from build123d import *

# Parameters (mm, degrees)
SKETCH001_R      = 2.5
PAD_DEPTH        = 10
HOLE_D           = 2.2
HOLE_DEPTH       = 25
HOLE_CBORE_D     = 4
HOLE_CBORE_DEPTH = 1.2


with BuildPart() as part:
    # Sketch001 → Pad (new body)
    with BuildSketch(Plane.XY):
        with BuildLine():
            Line((0, 0), (80, 0))
            Line((80, 0), (90, 5))
            Line((90, 5), (80, 10))
            Line((80, 10), (12.291288, 10))
            Line((12.291288, 5), (12.291288, 10))
            Line((2.5, 5), (12.291288, 5))
            ThreePointArc((2.291288, 6), (-2.447266, 4.489226), (2.5, 5))
            Line((11.291288, 6), (2.291288, 6))
            Line((11.291288, 10), (11.291288, 6))
            Line((0, 10), (11.291288, 10))
            ThreePointArc((0, 10), (-5, 5), (0, 0))
        make_face()
        with Locations((80, 5.087405)):
            Circle(SKETCH001_R, mode=Mode.SUBTRACT)
    extrude(amount=PAD_DEPTH)

    # Hole
    with Locations(Plane(origin=(0, 10, 0), x_dir=(-1, 0, 0), z_dir=(0, 1, 0))):
        with Locations((-6, 5)):
            CounterBoreHole(HOLE_D / 2, HOLE_CBORE_D / 2, HOLE_CBORE_DEPTH, depth=HOLE_DEPTH)


solid = part.part
Part model, mm, in its own coordinate system. A direction names the side the tool comes from. Give positions to 0.01 mm unless a question says otherwise; leave off trailing zeros. Order: outer loops, then holes, each group sorted by start corner. A loop starts at its lowest first (then second) coordinate and runs counter-clockwise, first axis right, second up. Notation, with made-up numbers: (-1, -31) - (25, -31) arc R13 cw to (25, -24) - close; hole circle Ø7 at (78.25, -21). An arc over 180 degrees is marked (long way). Use a Markdown table: item, result.
1) Probe L1, parallel to Y at x = 80, z = 2.25; L2, parallel to X at y = 7.25, z = 7.75; L3, parallel to X at y = 4, z = 0.5. List the from-to ranges inside material, lowest first. Write a range as from..to.
Checked values:
| item | result |
|---|---|
| L1 | 0..2.59, 7.59..10 |
| L2 | -4.47..-1.09, 1.09..11.29, 12.29..78.75, 81.25..85.5 |
| L3 | -4.9..-2.29, 2.29..77.75, 82.25..88 |
2) 3-axis set-ups, long thin cutter, end or side, ignore diameter. For faces 1 (the flat face through (84.93, 2.465, 4.93)), 2 (the flat face through (5, 8.8, 4)), 3 (the cylindrical face through (7.016, 2.465, 4.579)), 4 (the flat face through (11.291, 8, 5)), 5 (the flat face through (8, 6, 5)): which of +Z, -Z, +X, -X, +Y, -Y reach the whole face in a straight line?
Checked values:
| item | result |
|---|---|
| face 1 | +Z, -Z, +X, -Y |
| face 2 | +Y |
| face 3 | +Y, -Y |
| face 4 | +Z, -Z, +Y |
| face 5 | +Z, -Z |
3) Saw through at B-B on x = 6. List the corners of the cut face in (y, z).
Checked values:
| item | result |
|---|---|
| outline | (0, 0) - (5, 0) - (5, 3.9) - (0, 3.9) - close; (0, 6.1) - (5, 6.1) - (5, 10) - (0, 10) - close; (6, 0) - (10, 0) - (10, 3) - (8.8, 3) - (8.8, 3.9) - (6, 3.9) - close; (6, 6.1) - (8.8, 6.1) - (8.8, 7) - (10, 7) - (10, 10) - (6, 10) - close |
4) Saw through at C-C on z = 8.5. List the corners of the cut face in (x, y), plus the area to 3 significant figures.
Checked values:
| item | result |
|---|---|
| outline | (0, 0) - (80, 0) - (90, 5) - (80, 10) - (12.29, 10) - (12.29, 5) - (2.5, 5) arc R2.5 cw (long way) to (2.29, 6) - (11.29, 6) - (11.29, 10) - (0, 10) arc R5 ccw to start; hole circle Ø5 at (80, 5.09) |
| area | 836 mm² |
5) Saw through at A-A on z = 5. List the corners of the cut face in (x, y), plus the area to 3 significant figures.
Checked values:
| item | result |
|---|---|
| outline | (0, 0) - (4.9, 0) - (4.9, 5) - (2.5, 5) arc R2.5 cw (long way) to (2.29, 6) - (4.9, 6) - (4.9, 8.8) - (4, 8.8) - (4, 10) - (0, 10) arc R5 ccw to start; (7.1, 0) - (80, 0) - (90, 5) - (80, 10) - (12.29, 10) - (12.29, 5) - (7.1, 5) - close; (7.1, 6) - (11.29, 6) - (11.29, 10) - (8, 10) - (8, 8.8) - (7.1, 8.8) - close; hole circle Ø5 at (80, 5.09) |
| area | 814 mm² |
6) Flat gauge pins, fed straight in: P1, Ø2.5, axis at y = 8.5, z = 7, coming from the -X side; P2, Ø1.2, axis at y = 7.5, z = 7, coming from the +X side; P3, Ø1.5, axis at y = 7, z = 4, coming from the -X side; P4, Ø4.5, axis at x = 6, z = 5, coming from the +Y side. Where does each tip first touch, or does it go through?
Checked values:
| item | result |
|---|---|
| P1 | x = -4.47 |
| P2 | x = 86.2 |
| P3 | x = -4.84 |
| P4 | y = 10 |
7) Two-plate mould, pull along X, no slides. Class faces 6 (the cylindrical face through (78.016, 3.566, 4.93)), 7 (the cylindrical face through (-5, 5, 5)), 8 (the flat face through (42, 5, 10)): +X half, -X half, draft (parallel to the pull), parting line (faces both ways), or undercut.
Checked values:
| item | result |
|---|---|
| face 6 | undercut |
| face 7 | -X half |
| face 8 | draft |
